Work out the finished part from the listing and answer in its coordinate system (mm). Face numbers are marked on the shaded views. A direction names the side the tool comes from. Give positions to 0.01 mm unless a question says otherwise; leave off trailing zeros. Order: outer loops, then holes, each group sorted by start corner. A loop starts at its lowest first (then second) coordinate and runs counter-clockwise, first axis right, second up.
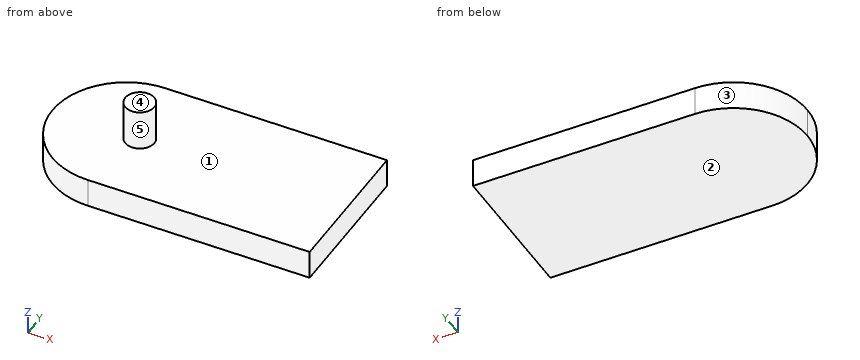
Autodesk Inventor part; units mm, degrees
ref_plane "YZ Plane" through (0, 0, 0) normal (1, 0, 0) x (0, 1, 0)
ref_plane "XZ Plane" through (0, 0, 0) normal (0, 1, 0) x (-1, 0, 0)
ref_plane "XY Plane" through (0, 0, 0) normal (0, 0, 1) x (1, 0, 0)
sketch "Sketch1" plane through (0, 0, 0) normal (0, 0, 1) x (1, 0, 0)
  line L0 (0, 0) -> (50.8, 0)
  line L1 (50.8, 0) -> (50.8, 25.4)
  line L2 (50.8, 25.4) -> (0, 25.4)
  line L3 (0, 25.4) -> (0, 0)
  dimension "d0" = 50.8
  dimension "d1" = 25.4
extrude "Extrusion1" add sketch "Sketch1" along normal blind 5
sketch "Sketch2" plane through (0, 0, 5) normal (0, 0, 1) x (1, 0, 0)
  circle A0 centre (15, 12.7) radius 2.5
  line L0 (0, 25.4) -> (0, 0)
  line L1 (50.8, 0) -> (50.8, 25.4)
  point P0 (50.8, 12.7)
  dimension "d4" = 5
  dimension "d5" = 15
extrude "Extrusion2" add sketch "Sketch2" along normal blind 7
full round fillet "Fillet1" first side at (16.9333, 0, 1.6667) centre faces at (0, 16.9333, 3.3333) second side at (33.8667, 25.4, 1.6667)
properties part number "Tilt_Camera_Side_Plate_2"
1. Given P1, Ø2, axis at x = 11, y = 19.5, coming from the +Z side; P2, Ø1.5, axis at x = 35.5, y = 21.5, coming from the -Z side; P3, Ø6, axis at y = 6, z = 1.5, coming from the -X side, each flat-ended and moving along its own axis, determine where each tip first touches the part or whether it passes through.
Findings below:
P1: stops at z = 5
P2: stops at z = 0
P3: stops at x = 0.55
2. The part is cut by section C-C (y = 3). Write down the section's boundary in (x, z), then the cut area to 3 significant figures.
Findings below:
outline: (4.5, 0) - (50.8, 0) - (50.8, 5) - (4.5, 5) - close
area: 231 mm2
3. Which of the six approach directions +Z, -Z, +X, -X, +Y, -Y give full straight-line access (tool end or side, diameter ignored) to the marked faces 4 and 5?
Findings below:
face 4: +Z, +X, -X, +Y, -Y
face 5: +Z
4. Straight lines are drawn through the part: probe 1 along X at (y, z) = (12.25, 2.5); probe 2 along Y at (x, z) = (15, 6.5); probe 3 along Z at (x, y) = (43, 1.25). For each, find the intervals that lie inside material, in ascending order.
Findings below:
probe 1: x = 0.01 to 50.8
probe 2: y = 10.2 to 15.2
probe 3: z = 0 to 5
5. The part is cut by section D-D (x = 36.5). Write down the section's boundary in (y, z).
Findings below:
outline: (0, 0) - (25.4, 0) - (25.4, 5) - (0, 5) - close
6. The part is cut by section A-A (x = 15). Write down the section's boundary in (y, z).
Findings below:
outline: (0, 0) - (25.4, 0) - (25.4, 5) - (15.2, 5) - (15.2, 12) - (10.2, 12) - (10.2, 5) - (0, 5) - close
7. The mould has two halves that part along Z. Classify the marked faces 1, 2 and 3: pulls with the +Z half, pulls with the -Z half, needs draft (parallel to the pull), parting line crosses it, or undercut.
Findings below:
face 1: pulls with the +Z half
face 2: pulls with the -Z half
face 3: needs draft
